Could you check a few things on this model? Use its own coordinates, in mm. Face numbers are marked on the shaded views. A direction names the side the tool comes from. Give positions to 0.01 mm unless a question says otherwise; leave off trailing zeros. Loops run counter-clockwise (first coordinate to the right, second up) from the corner with the lowest first, then second, coordinate; pieces in that order, holes last. Notation, with made-up numbers: (-28.75, 22) -> (14.25, 22) arc R17 cw to (14.25, 31) -> close; hole circle Ø4 at (16.25, 9.25). An arc over 180 degrees is marked (long way). Write each question's results on one line, items separated by ' | '. Start each with the question number.
Q1. If we section it at C-C, the plane z = 9.75: List the corners of the cut face in (x, y) for me, plus the area to 3 significant figures.
Q2. If we section it at B-B, the plane y = 0: List the corners of the cut face in (x, z) for me, plus the area to 3 significant figures.
Q3. If we section it at D-D, the plane x = 6.75: List the corners of the cut face in (y, z) for me.
Q4. If we section it at A-A, the plane x = 9.5: List the corners of the cut face in (y, z) for me.
Q5. Will these pins go through, and if not, where does the flat tip stop? P1, Ø4, axis at x = -3.5, y = 6, coming from the -Z side; P2, Ø1.1, axis at y = 4.5, z = 18, coming from the +X side; P3, Ø1.6, axis at x = 5, y = -2, coming from the +Z side.
Q6. If I drill on line 1 along Y through (x, z) = (3.5, 7.75); line 2 along X through (y, z) = (-7, 2.75); line 3 along X through (y, z) = (10, 10.25), over which ranges is the centre line in solid material (lowest first)?
Q7. We'd pull the mould along Z, two halves only. Please class the marked faces 3, 4 and 5: released by +Z, released by -Z, zero draft, split by the parting line, or undercut.
Q8. Which directions (+Z, -Z, +X, -X, +Y, -Y) give clear straight access to the entire face, cutting with the end or side of a thin tool? Please do the marked faces 1 and 2.
Autodesk Inventor part; units mm, degrees
ref_plane "YZ Plane" through (0, 0, 0) normal (1, 0, 0) x (0, 1, 0)
ref_plane "XZ Plane" through (0, 0, 0) normal (0, 1, 0) x (-1, 0, 0)
ref_plane "XY Plane" through (0, 0, 0) normal (0, 0, 1) x (1, 0, 0)
sketch "Sketch2" plane through (0, 0, 0) normal (0, 1, 0) x (-1, 0, 0)
  line L0 (0, 18.2) -> (0, 0)
  line L1 (0, 0) -> (-11, 0)
  line L2 (-11, 0) -> (-16, 2.5)
  line L3 (-16, 2.5) -> (-16, 11.2)
  line L4 (-16, 11.2) -> (-2.5, 11.2)
  line L5 (-2.5, 11.2) -> (-2.5, 18.2)
  line L6 (-2.5, 18.2) -> (0, 18.2)
  dimension "d0" = 18.2
  dimension "d1" = 11.2
  dimension "d2" = 2.5
  dimension "d3" = 16
  dimension "d4" = 5
  dimension "d5" = 2.5
extrude "Extrusion1" add sketch "Sketch2" along normal mid plane 38
fillet "Fillet1" radius 6 1 edges at (2.5, 0, 11.2)
sketch "Sketch3" plane through (0, -19, 18.2) normal (-1, 0, 0) x (0, 0, 1)
  line L0 (-9.7, 35.9) -> (-16.2, 35.9)
  line L1 (-16.2, 35.9) -> (-16.2, 2.1)
  line L2 (-16.2, 2.1) -> (-9.7, 2.1)
  line L3 (-9.7, 2.1) -> (-9.7, 35.9)
  line L4 (-18.2, 19) -> (-16.2, 19) construction
  line L5 (-18.2, 38) -> (-18.2, 0) construction
  line L6 (0, 0) -> (-18.2, 0) construction
  line L7 (-18.2, 38) -> (0, 38) construction
  dimension "d9" = 2
  dimension "d10" = 33.8
  dimension "d11" = 6.5
extrude "Extrusion2" cut sketch "Sketch3" against normal blind 10
sketch "Sketch4" plane through (0, -19, 18.2) normal (-1, 0, 0) x (0, 0, 1)
  circle A0 centre (-7.2, 19) radius 2
  line L0 (-7.2, 19) -> (-18.2, 19) construction
  dimension "d14" = 4
  dimension "d15" = 11
extrude "Extrusion3" add sketch "Sketch4" along normal blind 6.4
sketch "Sketch5" plane through (0, -19, 18.2) normal (-1, 0, 0) x (0, 0, 1)
  line L0 (-9.7, 21.5) -> (-11.7, 21.5)
  line L1 (-11.7, 16.5) -> (-9.7, 16.5)
  line L2 (-9.7, 16.5) -> (-9.7, 21.5)
  line L3 (-16.2, 35.9) -> (-9.7, 35.9) construction
  line L4 (-9.7, 2.1) -> (-16.2, 2.1) construction
  line L5 (-9.7, 35.9) -> (-9.7, 2.1) construction
  line L6 (-12.95, 35.9) -> (-12.95, 2.1) construction
  line L7 (-18.2, 19) -> (-9.9, 19)
  line L8 (-11.7, 18.5) -> (-9.9, 18.5)
  line L9 (-9.9, 18.5) -> (-9.9, 19.5)
  line L10 (-9.9, 19.5) -> (-11.7, 19.5)
  line L11 (-11.7, 21.5) -> (-11.7, 19.5)
  line L12 (-11.7, 18.5) -> (-11.7, 16.5)
  line L13 (-16.2, 21.5) -> (-14.2, 21.5)
  line L14 (-14.2, 16.5) -> (-16.2, 16.5)
  line L15 (-16.2, 16.5) -> (-16.2, 21.5)
  line L16 (-14.2, 18.5) -> (-16, 18.5)
  line L17 (-16, 18.5) -> (-16, 19.5)
  line L18 (-16, 19.5) -> (-14.2, 19.5)
  line L19 (-14.2, 21.5) -> (-14.2, 19.5)
  line L20 (-14.2, 18.5) -> (-14.2, 16.5)
  point P0 (-16, 19)
  dimension "d19" = 5
  dimension "d20" = 2
  dimension "d21" = 2.5
  dimension "d22" = 1
  dimension "d23" = 1.8
extrude "Extrusion4" add sketch "Sketch5" against normal up to next
properties part number "Boton de extraccion" material "ABS Plastic"
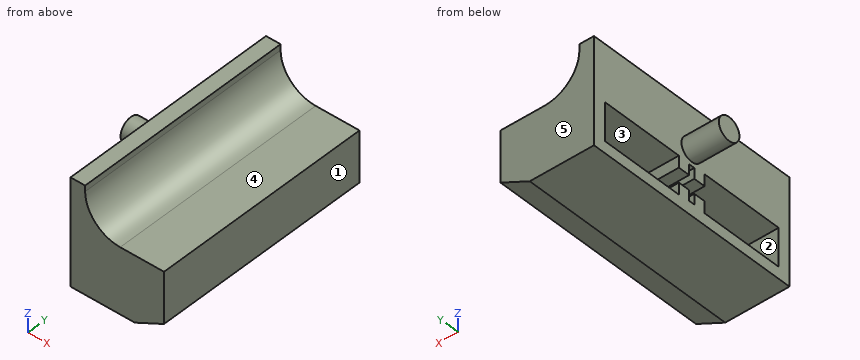
Final values:
1) outline: (-6.4, -1.56) -> (0, -1.56) -> (0, -19) -> (16, -19) -> (16, 19) -> (0, 19) -> (0, 1.56) -> (-6.4, 1.56) -> close | area: 628 mm²
2) outline: (-6.4, 9) -> (0, 9) -> (0, 8.3) -> (10, 8.3) -> (10, 2.2) -> (0, 2.2) -> (0, 0) -> (11, 0) -> (16, 2.5) -> (16, 11.2) -> (8.5, 11.2) arc R6 cw to (2.5, 17.2) -> (2.5, 18.2) -> (0, 18.2) -> (0, 13) -> (-6.4, 13) -> close | area: 163 mm²
3) outline: (-19, 0) -> (19, 0) -> (19, 11.46) -> (-19, 11.46) -> close; hole (-16.9, 2) -> (-2.5, 2) -> (-2.5, 4) -> (-0.5, 4) -> (-0.5, 2.2) -> (0.5, 2.2) -> (0.5, 4) -> (2.5, 4) -> (2.5, 2) -> (16.9, 2) -> (16.9, 8.5) -> (2.5, 8.5) -> (2.5, 6.5) -> (0.5, 6.5) -> (0.5, 8.3) -> (-0.5, 8.3) -> (-0.5, 6.5) -> (-2.5, 6.5) -> (-2.5, 8.5) -> (-16.9, 8.5) -> close
4) outline: (-19, 0) -> (19, 0) -> (19, 11.2) -> (-19, 11.2) -> close; hole (-16.9, 2) -> (-2.5, 2) -> (-2.5, 4) -> (-0.5, 4) -> (-0.5, 2.2) -> (0.5, 2.2) -> (0.5, 4) -> (2.5, 4) -> (2.5, 2) -> (16.9, 2) -> (16.9, 8.5) -> (2.5, 8.5) -> (2.5, 6.5) -> (0.5, 6.5) -> (0.5, 8.3) -> (-0.5, 8.3) -> (-0.5, 6.5) -> (-2.5, 6.5) -> (-2.5, 8.5) -> (-16.9, 8.5) -> close
5) P1: passes through | P2: stops at x = 2.5 | P3: stops at z = 13.02
6) line 1: y = -19 to -16.9, -2.5 to -0.5, 0.5 to 2.5, 16.9 to 19 | line 2: x = 10 to 16 | line 3: x = 0 to 16
7) face 3: undercut | face 4: released by +Z | face 5: zero draft
8) face 1: +Z, -Z, +X, +Y, -Y | face 2: -X
